Design review of the part built by this model. Coordinates are the model's own, in mm. Face numbers are marked on the shaded views. A direction names the side the tool comes from. Round coordinates to 2 decimals unless told otherwise and drop trailing zeros. Write each loop counter-clockwise with the first axis right and the second up, starting at its lowest first coordinate (ties: lowest second). Pieces come first, ordered by that corner, then holes.
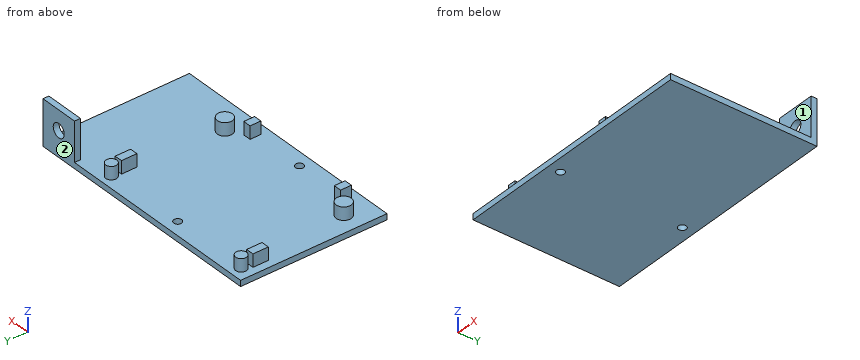
Autodesk Fusion 360 part; units mm, degrees
sketch "Sketch1" plane through (0, 0, 0) normal (0, 0, 1) x (1, 0, 0)
  line L0 (-47.74, 37.25) -> (47.74, 37.25)
  line L1 (47.74, 37.25) -> (47.74, -37.25)
  line L2 (47.74, -37.25) -> (-47.74, -37.25)
  line L3 (-47.74, -37.25) -> (-47.74, 37.25)
  line L4 (-47.74, 37.25) -> (47.74, -37.25) construction
  line L5 (47.74, 37.25) -> (-47.74, -37.25) construction
  circle A0 centre (41.24, 31.75) radius 2.78
  circle A1 centre (-41.24, 31.75) radius 2.78
  circle A2 centre (37.74, -23.25) radius 3.84
  circle A3 centre (-37.74, -23.25) radius 3.84
  line L6 (-30.74, -27.25) -> (-26.74, -27.25)
  line L7 (-26.74, -27.25) -> (-26.74, -33.25)
  line L8 (-26.74, -33.25) -> (-30.74, -33.25)
  line L9 (-30.74, -33.25) -> (-30.74, -27.25)
  line L10 (26.74, -27.25) -> (30.74, -27.25)
  line L11 (30.74, -27.25) -> (30.74, -33.25)
  line L12 (30.74, -33.25) -> (26.74, -33.25)
  line L13 (26.74, -33.25) -> (26.74, -27.25)
  line L14 (39.74, 27.75) -> (43.74, 27.75)
  line L15 (43.74, 27.75) -> (43.74, 19.95)
  line L16 (43.74, 19.95) -> (39.74, 19.95)
  line L17 (39.74, 19.95) -> (39.74, 27.75)
  line L18 (-43.74, 27.75) -> (-39.74, 27.75)
  line L19 (-39.74, 27.75) -> (-39.74, 19.95)
  line L20 (-39.74, 19.95) -> (-43.74, 19.95)
  line L21 (-43.74, 19.95) -> (-43.74, 27.75)
  point P0 (40, 20)
  dimension "d2" = 95.48
  dimension "d3" = 74.5
  dimension "d4" = 5.56
  dimension "d5" = 5.56
  dimension "d6" = 7.68
  dimension "d7" = 7.68
  dimension "d8" = 5.5
  dimension "d9" = 6.5
  dimension "d10" = 6.5
  dimension "d11" = 5.5
  dimension "d12" = 14
  dimension "d13" = 10
  dimension "d14" = 10
  dimension "d15" = 14
  dimension "d22" = 4
  dimension "d23" = 6
  dimension "d24" = 4
  dimension "d25" = 7
  dimension "d26" = 4
  dimension "d27" = 6
  dimension "d28" = 7
  dimension "d29" = 4
  dimension "d30" = 4
  dimension "d31" = 7.8
  dimension "d32" = 4
  dimension "d33" = 4
  dimension "d34" = 4
  dimension "d35" = 7.8
  dimension "d36" = 4
  dimension "d37" = 4
extrude "Extrude1" add sketch "Sketch1" along normal blind 9.5 contours A0 | A1 | A2 | A3 | L6 L7 L8 L9 | L10 L11 L12 L13 | L14 L15 L16 L17 | L18 L19 L20 L21 makes body 1 at (41.5609, -23.6323, 6.3333) makes body 2 at (-33.9191, -23.6323, 6.3333) makes body 3 at (30.74, -29.25, 3.1667) makes body 4 at (-26.74, -29.25, 3.1667) makes body 5 at (44.0062, 31.4732, 6.3333) makes body 6 at (-38.4738, 31.4732, 6.3333) makes body 7 at (43.74, 25.15, 3.1667) makes body 8 at (-39.74, 25.15, 6.3333)
extrude "Extrude2" add sketch "Sketch1" along normal blind 3 bodies 1 2 3 4 5 6 7 8
sketch "Sketch6" plane through (0, 0, 3) normal (0, 0, 1) x (-1, 0, 0)
  circle A0 centre (41.24, -31.75) radius 2.78
  circle A1 centre (37.74, 23.25) radius 3.84
  line L0 (26.74, 33.25) -> (30.74, 33.25)
  line L1 (30.74, 33.25) -> (30.74, 27.25)
  line L2 (30.74, 27.25) -> (26.74, 27.25)
  line L3 (26.74, 27.25) -> (26.74, 33.25)
  circle A2 centre (-37.74, 23.25) radius 3.84
  line L4 (-30.74, 33.25) -> (-26.74, 33.25)
  line L5 (-26.74, 33.25) -> (-26.74, 27.25)
  line L6 (-26.74, 27.25) -> (-30.74, 27.25)
  line L7 (-30.74, 27.25) -> (-30.74, 33.25)
  line L8 (-43.74, -19.95) -> (-39.74, -19.95)
  line L9 (-39.74, -19.95) -> (-39.74, -27.75)
  line L10 (-39.74, -27.75) -> (-43.74, -27.75)
  line L11 (-43.74, -27.75) -> (-43.74, -19.95)
  circle A3 centre (-41.24, -31.75) radius 2.78
  line L12 (39.74, -19.95) -> (43.74, -19.95)
  line L13 (43.74, -19.95) -> (43.74, -27.75)
  line L14 (43.74, -27.75) -> (39.74, -27.75)
  line L15 (39.74, -27.75) -> (39.74, -19.95)
  line L16 (47.74, 37.25) -> (-47.74, 37.25)
  line L17 (-47.74, 37.25) -> (-47.74, -37.25)
  line L18 (-47.74, -37.25) -> (47.74, -37.25)
  line L19 (47.74, -37.25) -> (47.74, 37.25)
  line L20 (-145.7882, -27) -> (145.7882, -27)
  line L21 (145.7882, -27) -> (145.7882, 27)
  line L22 (145.7882, 27) -> (-145.7882, 27)
  line L23 (-145.7882, 27) -> (-145.7882, -27)
  line L24 (-145.7882, -27) -> (145.7882, 27) construction
  line L25 (145.7882, -27) -> (-145.7882, 27) construction
  circle A4 centre (0, -31) radius 2
  line L26 (-20, 0) -> (-2.5, 0)
  circle A5 centre (0, 31) radius 2
  point P0 (0, -31)
  dimension "d42" = 54
  dimension "d44" = 4
  dimension "d47" = 4
  dimension "d50" = 31
move_face "OffsetFaces1" offset -0.5 2 faces at (-28.0733, -33.25, 5.1667) (29.4067, -33.25, 5.1667) on bodies 1
extrude "Extrude3" cut sketch "Sketch6" against normal blind 5 contours A4 | A5 bodies 1
extrude "Extrude5" add 1 faces at (47.74, 12.4167, 1) along direction (1, 0, 0) blind 30 on bodies 1 bodies 1
sketch "Sketch11" plane through (0, 37.25, 0) normal (0, 1, 0) x (-1, 0, 0)
  line L0 (-77.74, 0) -> (47.74, 0)
  line L1 (47.74, 0) -> (47.74, 3)
  line L2 (47.74, 3) -> (-77.74, 3)
  line L3 (-77.74, 3) -> (-77.74, 0)
  line L4 (-77.74, 3) -> (-57.74, 3)
  line L5 (-57.74, 3) -> (-57.74, 23)
  line L6 (-57.74, 23) -> (-77.74, 23)
  line L7 (-77.74, 23) -> (-77.74, 3)
  circle A0 centre (-67.74, 13) radius 3.5
  dimension "d56" = 20
  dimension "d57" = 20
  dimension "d58" = 7
  dimension "d59" = 10
  dimension "d60" = 10
extrude "Extrude6" add sketch "Sketch11" against normal blind 3 contours L2 L4 L5 L6 L7 bodies 1
1) For P1, Ø3, axis at x = 41.5, y = 32.5, coming from the +Z side; P2, Ø3, axis at y = -29.5, z = 7.5, coming from the -X side; P3, Ø3, axis at y = 22, z = 6.5, coming from the +X side, all flat-tipped, find the tip position at first contact; note any pin that passes through.
2) Add section C-C on x = 67.74. State the section outline as (y, z) points, and give its area (4 significant figures).
3) Add section B-B on x = 0. State the section outline as (y, z) points, and give its area (4 significant figures).
4) For line 1 along Y through (x, z) = (0, 2.3); line 2 along X through (y, z) = (-31, 1.4); line 3 along Z through (x, y) = (67.74, 35.75), list the stretches that pass through material, from the lowest coordinate up.
5) Add section D-D on y = -31. State the section outline as (x, z) points, and give its area (3 significant figures).
6) For the marked faces 1 and 2, list the 3-axis set-ups (+Z, -Z, +X, -X, +Y, -Y) from which the entire face can be reached by the end or side of a thin tool; tool diameter is ignored.
7) Add section A-A on z = 13. State the section outline as (x, y) points.
Computed:
1. P1: stops at z = 9.5
1. P2: stops at x = -30.74
1. P3: stops at x = 43.74
2. outline: (-37.25, 0) - (37.25, 0) - (37.25, 9.5) - (34.25, 9.5) - (34.25, 3) - (-37.25, 3) - close; (34.25, 16.5) - (37.25, 16.5) - (37.25, 23) - (34.25, 23) - close
2. area: 262.5 mm2
3. outline: (-37.25, 0) - (-33, 0) - (-33, 3) - (-37.25, 3) - close; (-29, 0) - (29, 0) - (29, 3) - (-29, 3) - close; (33, 0) - (37.25, 0) - (37.25, 3) - (33, 3) - close
3. area: 199.5 mm2
4. line 1: y = -37.25 to -33, -29 to 29, 33 to 37.25
4. line 2: x = -47.74 to -2, 2 to 77.74
4. line 3: z = 0 to 9.5, 16.5 to 23
5. outline: (-47.74, 0) - (-2, 0) - (-2, 3) - (-26.74, 3) - (-26.74, 9.5) - (-30.74, 9.5) - (-30.74, 3) - (-47.74, 3) - close; (2, 0) - (77.74, 0) - (77.74, 3) - (30.74, 3) - (30.74, 9.5) - (26.74, 9.5) - (26.74, 3) - (2, 3) - close
5. area: 416 mm2
6. face 1: +Z, +X, -Y
6. face 2: +Z, -Z, +X, -X, +Y
7. outline: (57.74, 34.25) - (64.24, 34.25) - (64.24, 37.25) - (57.74, 37.25) - close; (71.24, 34.25) - (77.74, 34.25) - (77.74, 37.25) - (71.24, 37.25) - close
